from build123d import *

# Parameters (mm, degrees)
SKETCH_1_R          = 4
EXTRUDE_1_DEPTH     = 14
SKETCH_2_OUTSIDE_W  = 13.6
SKETCH_2_OUTSIDE_H  = 13.6
SKETCH_2_OUTSIDE_R  = 3
CUT_EXTRUDE_1_DEPTH = 2


# Read off the part's stored shape, not the designer's step: M8 机械螺纹 螺柱1
with BuildPart() as part:
    # 草图1 → 凸台-拉伸1 (new body)
    with BuildSketch(Plane.XY):
        Circle(SKETCH_1_R)
    extrude(amount=-EXTRUDE_1_DEPTH)

    # 草图2 outside → 切除-拉伸1 (cut)
    with BuildSketch(Plane(origin=(0, 0, -14), x_dir=(-1, 0, 0), z_dir=(0, 0, -1))):
        Rectangle(SKETCH_2_OUTSIDE_W, SKETCH_2_OUTSIDE_H)
        Circle(SKETCH_2_OUTSIDE_R, mode=Mode.SUBTRACT)
    extrude(amount=-CUT_EXTRUDE_1_DEPTH, mode=Mode.SUBTRACT)

    # M8 机械螺纹 螺柱1 outline → M8 机械螺纹 螺柱1 (revolve, cut)
    with BuildSketch(Plane.XZ):
        Polygon((4, 0), (3.3235, 0), (4, -0.6765), align=None)
    revolve(axis=Axis((0, 0, 0), (0, 0, 1)), mode=Mode.SUBTRACT)

    # 草图4 one side → 旋转1 (revolve)
    with BuildSketch(Plane(origin=(0, 0, 0), x_dir=(0, 0, -1), z_dir=(1, 0, 0))):
        with BuildLine():
            Line((14, 6), (14, 0))
            Line((14, 0), (75.144445246, 0))
            ThreePointArc((75.144445246, 0), (74.809510044, 1.377472185), (73.879492165, 2.447368421))
            ThreePointArc((73.879492165, 2.447368421), (54.51207399, 9.769129661), (34.036579508, 6.693548387))
            ThreePointArc((34.036579508, 6.693548387), (26.766592165, 5.023444587), (19.371438197, 6))
            Line((19.371438197, 6), (14, 6))
        make_face()
    revolve(axis=Axis((0, 0, -14), (0, 0, -1)))


solid = part.part
Read the model definition and answer for the solid it produces. Units are mm, in the model's axes. A direction names the side the tool comes from. Give positions to 0.01 mm unless a question says otherwise; leave off trailing zeros. Write each loop counter-clockwise with the first axis right and the second up, starting at its lowest first coordinate (ties: lowest second). Pieces come first, ordered by that corner, then holes. Notation, with made-up numbers: (70, -10) - (123, -10) arc R35 cw to (123, 29) - close; hole circle Ø9 at (0, 43). An arc over 180 degrees is marked (long way). Use CSV: the item, a comma, the result in double quotes. Start each with the question number.
(1) For faces 1 (the flat face through (-1, 3, -12)), 2 (the cylindrical face through (0, -6, -17)), determine the directions among +Z, -Z, +X, -X, +Y, -Y from which every point of the face is accessible in a straight line to the end or side of a thin tool.
(2) Given P1, Ø5, axis at x = -2, z = -54, coming from the +Y side; P2, Ø4, axis at y = -6.5, z = -38.5, coming from the -X side; P3, Ø1.5, axis at y = -4, z = -9.5, coming from the -X side, each flat-ended and moving along its own axis, determine where each tip first touches the part or whether it passes through.
(3) Determine the mould class of faces 3 (the flat face through (0, 0, 0)), 4 (the cylindrical face through (-0.867, -3.905, -6.259)), 5 (the flat face through (-1, -3, -14)) for opening direction Z: +Z half, -Z half, draft (parallel to the pull), parting line (faces both ways), or undercut.
(4) Consider line 1 along Z through (x, y) = (2.25, -2.5); line 2 along Y through (x, z) = (1.5, -69.5); line 3 along Z through (x, y) = (-2.75, 0). Determine where each line is inside the solid, lowest interval first.
(5) Find section A-A (z = -16). Give the vertices of the cut face in (x, y).
Findings below:
1,face 1,"none"
1,face 2,"+Z"
2,P1,"y = 9.95"
2,P2,"x = -7.15"
2,P3,"x = -2.33"
3,face 3,"+Z half"
3,face 4,"draft"
3,face 5,"undercut"
4,line 1,"-72.53 to -14, -12 to -0.04"
4,line 2,"-4.93 to 4.93"
4,line 3,"-73.45 to 0"
5,outline,"circle Ø12 at (0, 0)"
